from build123d import *

# Parameters (mm, degrees)
F0_R           = 25
F0_W           = 32
F0_H           = 24
F1_DEPTH       = 20
F3_D           = 5
F3_CBORE_D     = 10
F3_CBORE_DEPTH = 5
F6_D           = 5.5
F7_R           = 5


with BuildPart() as f1:
    # F0 (on Top) → F1 (new body)
    with BuildSketch(Plane.XY):
        Circle(F0_R)
        Rectangle(F0_W, F0_H, mode=Mode.SUBTRACT)
    extrude(amount=F1_DEPTH)

    # F3 (through all)
    with Locations(Plane.XY.offset(20)):
        with Locations((0, 17.5), (0, -17.5)):
            CounterBoreHole(F3_D / 2, F3_CBORE_D / 2, F3_CBORE_DEPTH)

    # F6 (through all)
    with Locations(Plane(origin=(-34, 0, 0), x_dir=(0, -1, 0), z_dir=(-1, 0, 0))):
        with Locations((0, 10)):
            Hole(F6_D / 2)

    # F7
    f7_edges = [f1.edges().sort_by_distance(p)[0] for p in [
        (16, 12, 10),
        (-16, 12, 10),
        (-16, -12, 10),
        (16, -12, 10),
    ]]
    fillet(f7_edges, radius=F7_R)


solid = f1.part
Geometry check sheet. Reference: the model listing, model coordinates, mm. A direction names the side the tool comes from. Give positions to 0.01 mm unless a question says otherwise; leave off trailing zeros. Loops run counter-clockwise (first coordinate to the right, second up) from the corner with the lowest first, then second, coordinate; pieces in that order, holes last. Notation, with made-up numbers: M 42,2.5 L 100,2.5 A24 ccw 100,27.5 Z; hole C 38,-16.5 d6. An arc over 180 degrees is marked long. Write each question's results on one line, items separated by ' | '.
1) Release check for a two-part mould opening along Z. For faces 1 (the face through (16.3, 0.4, 0)), 2 (the face through (-1.08, 12.62, 17.54)), 3 (the face through (16.3, 0.4, 20)), 4 (the face through (-20.439, -0.358, 12.727)) record: +Z half, -Z half, draft (parallel to the pull), parting line (faces both ways), or undercut.
Answers follow:
face 1: -Z half | face 2: draft | face 3: +Z half | face 4: undercut
2) Thickness scan on line 1 (Y direction, x = 0, z = 18.8); line 2 (Z direction, x = 20.25, y = 0); line 3 (Y direction, x = 0, z = 5.75). Record the ranges inside material, lowest first.
Answers follow:
line 1: -25 to -22.5, -12.5 to -12, 12 to 12.5, 22.5 to 25 | line 2: 0 to 7.25, 12.75 to 20 | line 3: -25 to -20, -15 to -12, 12 to 15, 20 to 25
3) Gauge pin test, flat ends, axial feed: pin 1 (5 mm diameter, centred on x = -9.5, z = 16.5, fed in from +Y); pin 2 (4 mm diameter, centred on y = -7, z = 17, fed in from +X); pin 3 (4 mm diameter, centred on y = 14.5, z = 3.5, fed in from -X); pin 4 (4.5 mm diameter, centred on y = 0, z = 10, fed in from +X). Record the tip position at first contact, or that the pin passes through.
Answers follow:
pin 1: y = 24 | pin 2: x = 24.49 | pin 3: x = -21.65 | pin 4: through
4) Section check A-A, the plane y = 0. Record the boundary of the cut face in (x, z).
Answers follow:
outline: M -25,0 L -16,0 L -16,7.25 L -25,7.25 Z; M -25,12.75 L -16,12.75 L -16,20 L -25,20 Z; M 16,0 L 25,0 L 25,7.25 L 16,7.25 Z; M 16,12.75 L 25,12.75 L 25,20 L 16,20 Z
5) Section check B-B, the plane z = 10. Record the boundary of the cut face in (x, y), plus the area to 3 significant figures.
Answers follow:
outline: M -24.85,-2.75 A25 ccw 24.85,-2.75 L 16,-2.75 L 16,-7 A5 cw 11,-12 L -11,-12 A5 cw -16,-7 L -16,-2.75 Z; M -24.85,2.75 L -16,2.75 L -16,7 A5 cw -11,12 L 11,12 A5 cw 16,7 L 16,2.75 L 24.85,2.75 A25 ccw Z; hole C 0,-17.5 d5; hole C 0,17.5 d5 | area: 1,080 mm2
6) Tool access check on faces 5 (the face through (-16, -1.7, 7.6)), 6 (the face through (20.563, -0.358, 12.727)), 7 (the face through (1, 20, 15)). Record the directions out of +Z, -Z, +X, -X, +Y, -Y that give a thin tool (end or side, any length) a straight path to the whole face; none if there is none.
Answers follow:
face 5: +Z, -Z | face 6: +X, -X | face 7: +Z
7) Section check C-C, the plane x = 0. Record the boundary of the cut face in (y, z), plus the area to 3 significant figures.
Answers follow:
outline: M -25,0 L -20,0 L -20,15 L -22.5,15 L -22.5,20 L -25,20 Z; M -15,0 L -12,0 L -12,20 L -12.5,20 L -12.5,15 L -15,15 Z; M 12,0 L 15,0 L 15,15 L 12.5,15 L 12.5,20 L 12,20 Z; M 20,0 L 25,0 L 25,20 L 22.5,20 L 22.5,15 L 20,15 Z | area: 270 mm2
8) Section check D-D, the plane x = 6. Record the boundary of the cut face in (y, z).
Answers follow:
outline: M -24.27,0 L -12,0 L -12,20 L -24.27,20 Z; M 12,0 L 24.27,0 L 24.27,20 L 12,20 Z
